```python
from build123d import *

# Parameters (mm, degrees)
F0_R      = 12.5
F1_DEPTH  = 15
F3_DEPTH  = 15
F5_DEPTH  = 13
F10_R     = 3
F11_R     = 11.5
F12_DEPTH = 12.6699203183
F14_R     = 11.5
F15_DEPTH = 13


with BuildPart() as f1:
    # F0 (on Top) → F1 (new body)
    with BuildSketch(Plane.XY):
        Circle(F0_R)
    extrude(amount=-F1_DEPTH)

    # F2 (on Front) → F3 (cut, symmetric)
    with BuildSketch(Plane.XZ):
        Polygon((12.5, 0), (-12.5, 0), (12.5, -11.3443713635), align=None)
    extrude(amount=F3_DEPTH, both=True, mode=Mode.SUBTRACT)

    # F4 (on Right) → F5 (join)
    with BuildSketch(Plane.YZ):
        with BuildLine():
            add(Edge.make_bspline(
                [(4.1614882648, -4.4021867216), (2.3196844094, -4.4021867216), (3.2405863371, -9.0699917637), (4.1614882648, -13.7377968058), (5.0823901925, -9.0699917637), (6.0032921202, -4.4021867216), (4.1614882648, -4.4021867216)],
                knots=[0, 0, 0, 2.0943951024, 2.0943951024, 4.1887902048, 4.1887902048, 6.2831853072, 6.2831853072, 6.2831853072], degree=2, weights=[1, 0.5, 1, 0.5, 1, 0.5, 1]))
        make_face()
        with BuildLine():
            add(Edge.make_bspline(
                [(-4.1614882648, -4.4021867216), (-6.0032921202, -4.4021867216), (-5.0823901925, -9.0699917637), (-4.1614882648, -13.7377968058), (-3.2405863371, -9.0699917637), (-2.3196844094, -4.4021867216), (-4.1614882648, -4.4021867216)],
                knots=[0, 0, 0, 2.0943951024, 2.0943951024, 4.1887902048, 4.1887902048, 6.2831853072, 6.2831853072, 6.2831853072], degree=2, weights=[1, 0.5, 1, 0.5, 1, 0.5, 1]))
        make_face()
    extrude(amount=-F5_DEPTH)

    # F8 (on Front) → F9 (revolve)
    with BuildSketch(Plane.XZ):
        with BuildLine():
            Line((0, -5.6721856818), (18.2126128557, -13.9366114312))
            ThreePointArc((18.2126128557, -13.9366114312), (17.6536526203, 0.5365345313), (7.5079209485, 10.8732902815))
            Line((7.5079209485, 10.8732902815), (0, -5.6721856818))
        make_face()
    revolve(axis=Axis((3.7539604743, 0, 2.6005522999), (0.4132212875, 0, 0.9106306428)))

    # F10
    f10_edges = [f1.edges().sort_by_distance(p)[0] for p in [
        (-18.212613, 0, 2.59224),
    ]]
    fillet(f10_edges, radius=F10_R)

    # F11 (on Top) → F12 (cut, through all)
    with BuildSketch(Plane.XY):
        Circle(F11_R)
    extrude(amount=F12_DEPTH, mode=Mode.SUBTRACT)

    # F14 (on face) → F15 (cut)
    with BuildSketch(Plane.XY):
        Circle(F14_R)
    extrude(amount=-F15_DEPTH, mode=Mode.SUBTRACT)


solid = f1.part
```
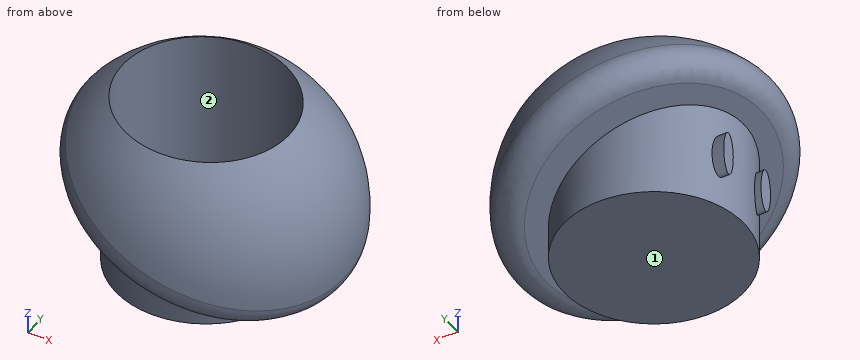
Model file for the job. Use its own axes, mm. Face numbers are marked on the shaded views. Give positions to 0.01 mm unless a question says otherwise; leave off trailing zeros. Order: outer loops, then holes, each group sorted by start corner. A loop starts at its lowest first (then second) coordinate and runs counter-clockwise, first axis right, second up.
1) Wall check: probe 1 along X at (y, z) = (-2, -12); probe 2 along Y at (x, z) = (0, -6.5); probe 3 along Z at (x, y) = (6, 3.5). Give the ranges that are in metal, low to high.
2) Pin check, flat tips, straight feed: pin 1 (3 mm diameter, centred on y = -12, z = 0.5, fed in from -X); pin 2 (7 mm diameter, centred on x = 2, y = -0.5, fed in from +Z); pin 3 (2 mm diameter, centred on y = 11, z = -8.5, fed in from +X). Stop position of each tip, or through.
3) Saw through at A-A, the plane z = 8. Write the cut outline in (x, y).
4) Mould opens along Y. For the marked faces 1 and 2 say: +Y half, -Y half, draft (parallel to the pull), parting line (faces both ways), or undercut.
Computed:
1. probe 1: x = -12.34 to -11.32, 11.32 to 12.34, 13.94 to 17.93
1. probe 2: y = -12.5 to -11.5, 11.5 to 12.5
1. probe 3: z = -15 to -13
2. pin 1: stops at x = -13.34
2. pin 2: stops at z = -13
2. pin 3: stops at x = 16.6
3. outline: circle Ø25.75 at (-0.79, 0); hole circle Ø23 at (0, 0)
4. face 1: draft
4. face 2: undercut
